Study the drawing (mm; zero at the part's minimum x, y, z) and answer. A direction names the side the tool comes from. Round coordinates to 2 decimals unless told otherwise and drop trailing zeros. Loops run counter-clockwise (first coordinate to the right, second up) from the corner with the lowest first, then second, coordinate; pieces in that order, holes last. Notation, with made-up numbers: (-28, 48) -> (19, 48) arc R19 ccw to (19, 82) -> close; hole circle Ø7 at (41, 68.25). An arc over 180 degrees is marked (long way). Answer in a Markdown table with one row per item. Add a question column.
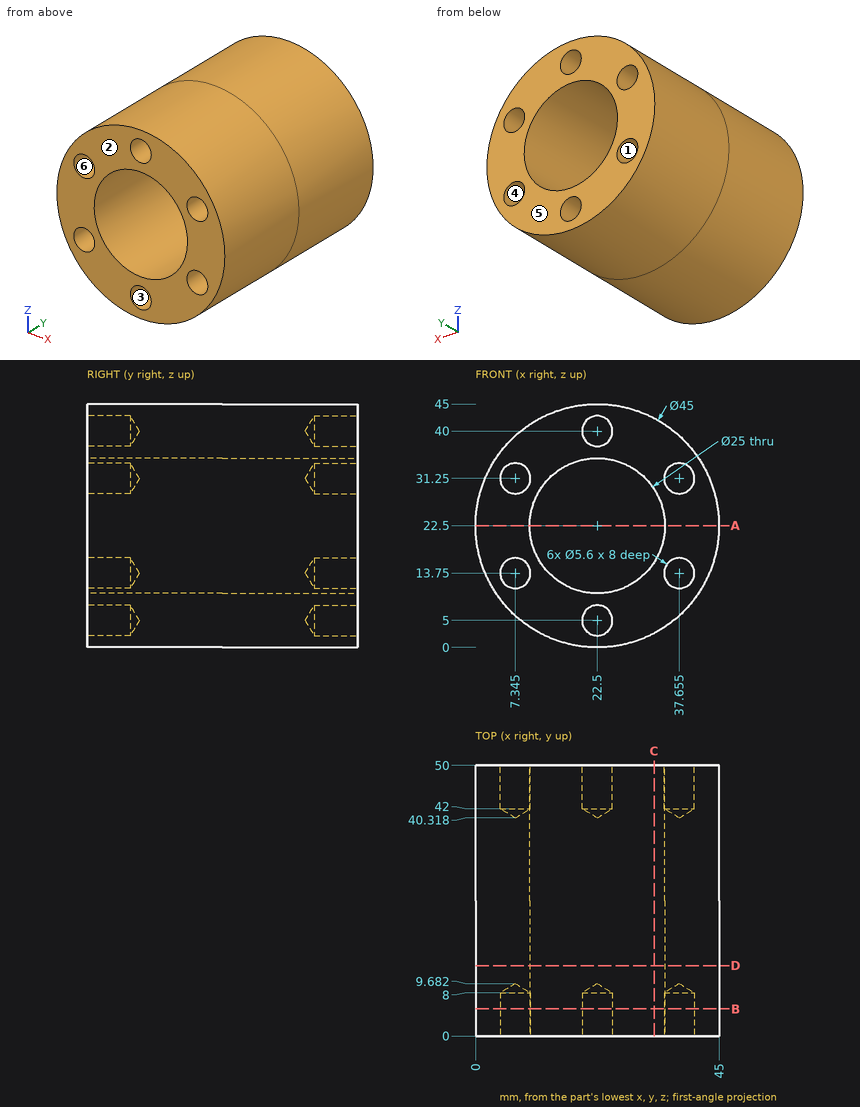
Item 1: The mould has two halves that part along Z. Classify the marked faces 4, 5 and 6: +Z half, -Z half, draft (parallel to the pull), parting line (faces both ways), or undercut.
Item 2: Section D-D, the plane y = 13 is taken. Write down the section's boundary in (x, z), and give its area (3 significant figures).
Item 3: Section B-B, the plane y = 5 is taken. Give the number of separate pieces and of enclosed holes in the cut face.
Item 4: Section C-C, the plane x = 33 is taken. Write down the section's boundary in (y, z), and give its area (3 significant figures).
Item 5: Consider L1, parallel to X at y = 46, z = 13.75 (1 decimal); L2, parallel to Z at x = 34, y = 41 (1 decimal); L3, parallel to X at y = 16.5, z = 22.5. Determine where each line is inside the solid, lowest interval first. Write a range as from..to.
Item 6: For the marked faces 1, 2 and 3, determine the directions among +Z, -Z, +X, -X, +Y, -Y from which every point of the face is accessible in a straight line to the end or side of a thin tool.
Item 7: Section A-A, the plane z = 22.5 is taken. Write down the section's boundary in (x, y).
Item 8: Flat-ended cylindrical pins translate along their axes: P1, Ø12, axis at x = 15, y = 22.5, coming from the -Z side; P2, Ø4.5, axis at x = 22.5, z = 5, coming from the -Y side; P3, Ø3, axis at x = 21.5, y = 37, coming from the +Z side; P4, Ø4.5, axis at x = 7.34, z = 13.75, coming from the +Y side. Find the tip coordinate at first contact, or state that the pin passes through.
Here are the results:
| question | item | result |
|---|---|---|
| 1 | face 4 | undercut |
| 1 | face 5 | draft |
| 1 | face 6 | undercut |
| 2 | outline | circle Ø45 at (22.5, 22.5); hole circle Ø25 at (22.5, 22.5) |
| 2 | area | 1,100 mm² |
| 3 | separate pieces | 1 |
| 3 | enclosed holes | 7 |
| 4 | outline | (0, 2.6) -> (50, 2.6) -> (50, 15.72) -> (0, 15.72) -> close; (0, 29.28) -> (50, 29.28) -> (50, 42.4) -> (0, 42.4) -> close |
| 4 | area | 1,310 mm² |
| 5 | L1 | x = 1.8..4.5, 10.1..13.6, 31.4..34.9, 40.5..43.2 |
| 5 | L2 | z = 3.2..17.6, 27.4..41.8 |
| 5 | L3 | x = 0..10, 35..45 |
| 6 | face 1 | +Y |
| 6 | face 2 | +Z, -Z, +X, -X, -Y |
| 6 | face 3 | -Y |
| 7 | outline | (0, 0) -> (10, 0) -> (10, 50) -> (0, 50) -> close; (35, 0) -> (45, 0) -> (45, 50) -> (35, 50) -> close |
| 8 | P1 | stops at z = 0.05 |
| 8 | P2 | stops at y = 8.33 |
| 8 | P3 | stops at z = 45 |
| 8 | P4 | stops at y = 41.67 |
